from build123d import *

# Parameters (mm, degrees)
BOSS_EXTRUDE1_DEPTH = 8
CHAMFER1_SIZE       = 3
SKETCH3_R           = 3.25
CUT_EXTRUDE2_DEPTH  = 19
SKETCH4_R           = 17
BOSS_EXTRUDE2_DEPTH = 3
SKETCH5_R           = 17
SKETCH5_R_2         = 15
BOSS_EXTRUDE3_DEPTH = 2
SKETCH6_R           = 8
BOSS_EXTRUDE4_DEPTH = 6.5
SKETCH7_R           = 8
BOSS_EXTRUDE5_DEPTH = 3
SKETCH8_R           = 6
CUT_EXTRUDE3_DEPTH  = 23
BOSS_EXTRUDE6_REACH = 39
SKETCH9_W           = 34
SKETCH9_H           = 2
CUT_EXTRUDE4_DEPTH  = 2
SKETCH11_W          = 2
SKETCH11_H          = 2
CUT_REVOLVE1_ANGLE  = 180
SKETCH12_R          = 2
CUT_EXTRUDE5_DEPTH  = 12
SKETCH13_R          = 2
CUT_EXTRUDE6_DEPTH  = 4


with BuildPart() as part:
    # Sketch1 → Boss-Extrude1 (new body, symmetric)
    with BuildSketch(Plane.XY):
        with BuildLine():
            Line((-35.5, 3), (-19, 3))
            Line((-19, 3), (-19, 16))
            ThreePointArc((-19, 16), (0, 35), (19, 16))
            Line((19, 16), (19, 3))
            Line((19, 3), (35.5, 3))
            Line((35.5, 3), (35.5, -3))
            Line((35.5, -3), (17, -3))
            Line((17, -3), (17, 16))
            ThreePointArc((17, 16), (0, 33), (-17, 16))
            Line((-17, 16), (-17, -3))
            Line((-17, -3), (-35.5, -3))
            Line((-35.5, -3), (-35.5, 3))
        make_face()
    extrude(amount=BOSS_EXTRUDE1_DEPTH, both=True)

    # Chamfer1
    chamfer1_edges = [part.edges().sort_by_distance(p)[0] for p in [
        (-35.5, 0, -8),
        (35.5, 0, -8),
        (-35.5, 0, 8),
        (35.5, 0, 8),
    ]]
    chamfer(chamfer1_edges, length=CHAMFER1_SIZE)

    # Sketch3 → Cut-Extrude2 (cut)
    with BuildSketch(Plane(origin=(0, 3, 0), x_dir=(1, 0, 0), z_dir=(0, 1, 0))):
        with Locations((28, 0)):
            Circle(SKETCH3_R)
        with Locations((-28, 0)):
            Circle(SKETCH3_R)
    extrude(amount=-CUT_EXTRUDE2_DEPTH, mode=Mode.SUBTRACT)

    # Sketch4 → Boss-Extrude2 (add, symmetric)
    with BuildSketch(Plane.XY):
        with Locations((0, 16)):
            Circle(SKETCH4_R)
    extrude(amount=BOSS_EXTRUDE2_DEPTH, both=True)

    # Sketch5 → Boss-Extrude3 (add)
    with BuildSketch(Plane.XY.offset(3)):
        with Locations((0, 16)):
            Circle(SKETCH5_R)
        with Locations((0, 16)):
            Circle(SKETCH5_R_2, mode=Mode.SUBTRACT)
    boss_extrude3 = extrude(amount=BOSS_EXTRUDE3_DEPTH)

    # Mirror1: Boss-Extrude3 across plane
    add(boss_extrude3.mirror(Plane.XY))

    # Sketch6 → Boss-Extrude4 (add)
    with BuildSketch(Plane.XY.offset(3)):
        with Locations((0, 16)):
            Circle(SKETCH6_R)
    extrude(amount=BOSS_EXTRUDE4_DEPTH)

    # Sketch7 → Boss-Extrude5 (add)
    with BuildSketch(Plane(origin=(0, 0, -3), x_dir=(-1, 0, 0), z_dir=(0, 0, -1))):
        with Locations((0, 16)):
            Circle(SKETCH7_R)
    extrude(amount=BOSS_EXTRUDE5_DEPTH)

    # Sketch8 → Cut-Extrude3 (cut)
    with BuildSketch(Plane.XY.offset(9.5)):
        with Locations((0, 16)):
            Circle(SKETCH8_R)
    extrude(amount=-CUT_EXTRUDE3_DEPTH, mode=Mode.SUBTRACT)

    # Sketch9 → Boss-Extrude6 (add, up to next)
    with BuildSketch(Plane(origin=(0, -2, 0), x_dir=(1, 0, 0), z_dir=(0, 1, 0)), mode=Mode.PRIVATE) as boss_extrude6_sk1:
        Rectangle(SKETCH9_W, SKETCH9_H)
    boss_extrude6_tool1 = extrude(boss_extrude6_sk1.sketch, amount=BOSS_EXTRUDE6_REACH, mode=Mode.PRIVATE) - part.part
    add(boss_extrude6_tool1.solids().sort_by_distance((0, -2, 0))[0])

    # Sketch10 → Cut-Extrude4 (cut)
    with BuildSketch(Plane(origin=(19, 0, 0), x_dir=(0, 0, -1), z_dir=(1, 0, 0))):
        Polygon((-8, 3), (-8, 16), (-6, 16), align=None)
        Polygon((6, 16), (8, 3), (8, 16), align=None)
    cut_extrude4 = extrude(amount=-CUT_EXTRUDE4_DEPTH, mode=Mode.SUBTRACT)

    # Mirror2: Cut-Extrude4 across plane
    add(cut_extrude4.mirror(Plane(origin=(0, 0, 0), x_dir=(0, 0, 1), z_dir=(1, 0, 0))), mode=Mode.SUBTRACT)

    # Sketch11 → Cut-Revolve1 (revolve, cut)
    with BuildSketch(Plane.XZ.offset(-16)):
        with Locations((-18, 7)):
            Rectangle(SKETCH11_W, SKETCH11_H)
        with Locations((-18, -7)):
            Rectangle(SKETCH11_W, SKETCH11_H)
    revolve(axis=Axis((0, 16, 3), (0, 0, -1)), revolution_arc=CUT_REVOLVE1_ANGLE, mode=Mode.SUBTRACT)

    # Sketch12 → Cut-Extrude5 (cut)
    with BuildSketch(Plane(origin=(0, 0, 0), x_dir=(0, 0, -1), z_dir=(1, 0, 0))):
        with Locations((-6.5, 16)):
            Circle(SKETCH12_R)
    extrude(amount=CUT_EXTRUDE5_DEPTH, mode=Mode.SUBTRACT)

    # Sketch13 → Cut-Extrude6 (cut)
    with BuildSketch(Plane(origin=(0, 20, 0), x_dir=(1, 0, 0), z_dir=(0, 1, 0))):
        with Locations((0, -6.5)):
            Circle(SKETCH13_R)
    extrude(amount=CUT_EXTRUDE6_DEPTH, mode=Mode.SUBTRACT)


solid = part.part
The model under review builds one solid part; all positions refer to its coordinate system, in mm. A direction names the side the tool comes from. Give positions to 0.01 mm unless a question says otherwise; leave off trailing zeros. Order: outer loops, then holes, each group sorted by start corner. A loop starts at its lowest first (then second) coordinate and runs counter-clockwise, first axis right, second up. Notation, with made-up numbers: (58.25, 6) -> (68.25, 6) arc R14 ccw to (68.25, 29) -> close; hole circle Ø10 at (80.25, 63.25). An arc over 180 degrees is marked (long way). Write item = value, one per line. Start each with the question number.
(1) Tool access review of faces 4 (the flat face through (-24, 3, 0)), 5 (the cylindrical face through (1.908, 22.812, 5.899)), 6 (the flat face through (18.014, 9.591, 6.986)): name each direction out of +Z, -Z, +X, -X, +Y, -Y from which nothing blocks a thin tool from reaching the whole face with its end or side.
(2) For L1, parallel to Z at x = 28, y = 0.7; L2, parallel to Y at x = 0, z = -3.45; L3, parallel to X at y = 7, z = -6.5, list the stretches that pass through material, from the lowest coordinate up. Write a range as from..to.
(3) Take a section at B-B (x = -28). Write out the cut boundary in (y, z), plus the area to 3 significant figures.
(4) Draft analysis for pull direction Z (two halves, no side actions). For faces 1 (the cylindrical face through (0.374, 32.996, -5.493)), 2 (the flat face through (-2, 22, 9.5)), 3 (the cylindrical face through (-24.9, 0.04, -0.98)), state which applies: +Z half, -Z half, draft (parallel to the pull), parting line (faces both ways), or undercut.
(5) Take a section at A-A (z = 0). Write out the cut boundary in (x, y), plus the area to 3 significant figures.
(6) For pin 1 Ø1.6 at (x, z) = (4, 0.5) entering from -Y; pin 2 Ø5 at (y, z) = (16, 6.5) entering from -X; pin 3 Ø10 at (y, z) = (18.5, -3) entering from +X, all flat-tipped, find the tip position at first contact; note any pin that passes through.
(7) Take a section at C-C (x = 11). Write out the cut boundary in (y, z).
(8) Take a section at D-D (y = 26). Write out the cut boundary in (x, z), plus the area to 3 significant figures.
Returned:
q1.face_4 = +Z, -Z, -X, +Y
q1.face_5 = none
q1.face_6 = +Z, +X, +Y
q2.L1 = -8..-3.25, 3.25..8
q2.L2 = -1..1, 8..10, 22..24, 31..35
q2.L3 = -19..-17, 17..19
q3.outline = (-3, -8) -> (3, -8) -> (3, -3.25) -> (-3, -3.25) -> close; (-3, 3.25) -> (3, 3.25) -> (3, 8) -> (-3, 8) -> close
q3.area = 57.0 mm²
q4.face_1 = draft
q4.face_2 = +Z half
q4.face_3 = undercut
q5.outline = (-35.5, -3) -> (-31.25, -3) -> (-31.25, 3) -> (-35.5, 3) -> close; (-24.75, -3) -> (-17, -3) -> (-17, -2) -> (17, -2) -> (17, -3) -> (24.75, -3) -> (24.75, 3) -> (19, 3) -> (19, 16) arc R19 ccw to (-19, 16) -> (-19, 3) -> (-24.75, 3) -> close; (31.25, -3) -> (35.5, -3) -> (35.5, 3) -> (31.25, 3) -> close; hole circle Ø12 at (0, 16)
q5.area = 1,260 mm²
q6.pin_1 = -2
q6.pin_2 = -19
q6.pin_3 = 19
q7.outline = (-2, -1) -> (3.04, -1) -> (3.04, -5) -> (5.8, -5) -> (5.8, -3) -> (26.2, -3) -> (26.2, -5) -> (28.96, -5) -> (28.96, -6) -> (31.49, -6) -> (31.49, 6) -> (28.96, 6) -> (28.96, 5) -> (26.2, 5) -> (26.2, 3) -> (5.8, 3) -> (5.8, 5) -> (3.04, 5) -> (3.04, 1) -> (-2, 1) -> close
q8.outline = (-16.16, -6) -> (-13.75, -6) -> (-13.75, -5) -> (-11.18, -5) -> (-11.18, -3) -> (11.18, -3) -> (11.18, -5) -> (13.75, -5) -> (13.75, -6) -> (16.16, -6) -> (16.16, 6) -> (13.75, 6) -> (13.75, 5) -> (11.18, 5) -> (11.18, 3) -> (-11.18, 3) -> (-11.18, 5) -> (-13.75, 5) -> (-13.75, 6) -> (-16.16, 6) -> close
q8.area = 243 mm²
